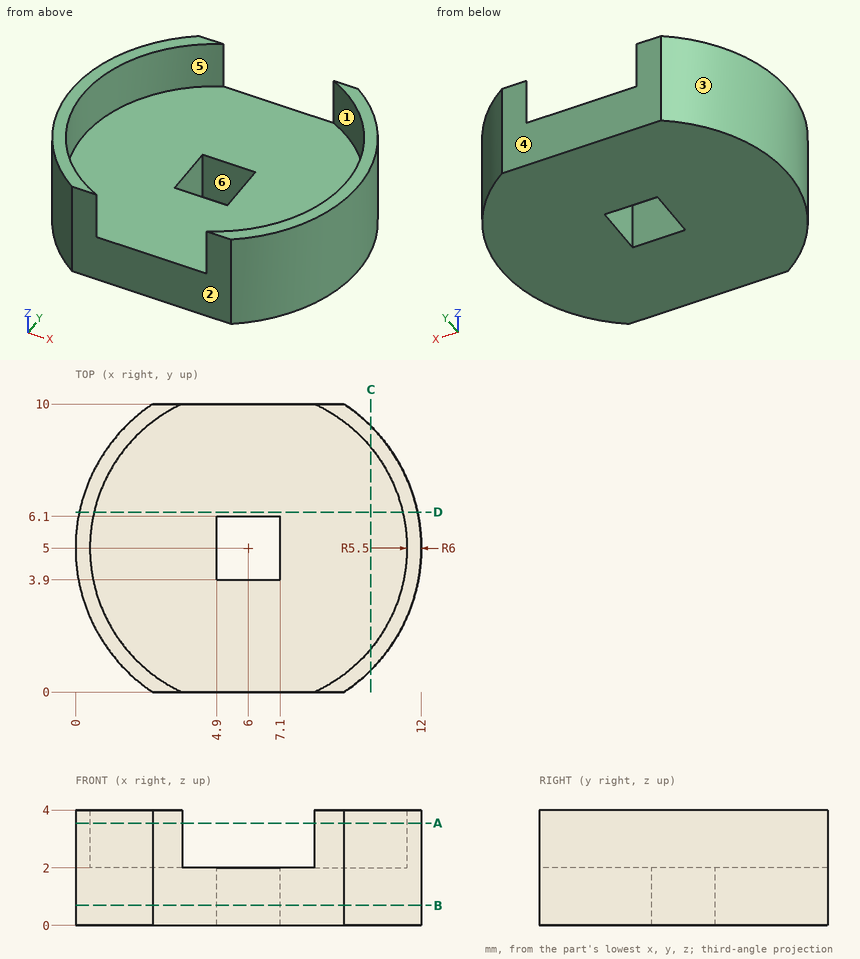
Source: three-view drawing plus pictorial views. Frame: mm from the lowest corner of the part. A direction names the side the tool comes from. Round coordinates to 2 decimals unless told otherwise and drop trailing zeros. Order: outer loops, then holes, each group sorted by start corner. A loop starts at its lowest first (then second) coordinate and runs counter-clockwise, first axis right, second up. Notation, with made-up numbers: (74.5, 54) -> (119.5, 54) arc R11 cw to (119.5, 63) -> close; hole circle Ø5 at (-30, -31). An arc over 180 degrees is marked (long way). Use CSV: the item, a comma, the result in double quotes. Start each with the question number.
1) Set-up query: the marked faces 4, 5 and 6. Return all of +Z, -Z, +X, -X, +Y, -Y with unobstructed straight access to the full face (end or side cutting, diameter ignored); none if empty.
2) Section C-C (x = 10.25). Return the cut outline in (y, z).
3) Draft query along X for the marked faces 1, 2 and 3. Return one class per face: +X half, -X half, draft (parallel to the pull), parting line (faces both ways), or undercut.
4) Section A-A (z = 3.55). Return the cut outline in (x, y).
5) Section D-D (y = 6.25). Return the cut outline in (x, z), and give its area (3 significant figures).
6) Section B-B (z = 0.7). Return the cut outline in (x, y).
7) First-contact query: pin 1 Ø6 at (x, y) = (8, 7) entering from -Z; pin 2 Ø2 at (y, z) = (2, 2) entering from +X; pin 3 Ø5 at (x, y) = (4, 4.5) entering from +Z. Flat tips, straight axial feed; report the tip coordinate or a pass-through.
8) Material intervals for line 1 along Y through (x, z) = (6, 1.2); line 2 along Z through (x, y) = (3, 8); line 3 along X through (y, z) = (2.75, 3.35), sorted ascending. Write a range as from..to.
Returned:
1,face 4,"+Z, -Z, +X, -X, +Y"
1,face 5,"+Z"
1,face 6,"+Z, -Z"
2,outline,"(0.76, 0) -> (9.24, 0) -> (9.24, 4) -> (8.49, 4) -> (8.49, 2) -> (1.51, 2) -> (1.51, 4) -> (0.76, 4) -> close"
3,face 1,"undercut"
3,face 2,"draft"
3,face 3,"-X half"
4,outline,"(2.68, 0) -> (3.71, 0) arc R5.5 cw to (3.71, 10) -> (2.68, 10) arc R6 ccw to start; (8.29, 0) -> (9.32, 0) arc R6 ccw to (9.32, 10) -> (8.29, 10) arc R5.5 cw to start"
5,outline,"(0.13, 0) -> (11.87, 0) -> (11.87, 4) -> (11.36, 4) -> (11.36, 2) -> (0.64, 2) -> (0.64, 4) -> (0.13, 4) -> close"
5,area,"25.5 mm²"
6,outline,"(2.68, 0) -> (9.32, 0) arc R6 ccw to (9.32, 10) -> (2.68, 10) arc R6 ccw to start; hole (4.9, 3.9) -> (7.1, 3.9) -> (7.1, 6.1) -> (4.9, 6.1) -> close"
7,pin 1,"stops at z = 0"
7,pin 2,"stops at x = 11.66"
7,pin 3,"stops at z = 2"
8,line 1,"y = 0..3.9, 6.1..10"
8,line 2,"z = 0..2"
8,line 3,"x = 0.44..0.98, 11.02..11.56"
